```python
from build123d import *

# Parameters (mm, degrees)
BOSS_EXTRUDE1_DEPTH       = 76.2
CUT_EXTRUDE1_REACH        = 112.716
SKETCH7_R                 = 3.175
TAP_DRILL_FOR_8_32_TAP2_D = 3.4544
TAP_DRILL_FOR_8_32_TAP4_D = 3.4544
TAP_DRILL_FOR_6_32_TAP1_D = 2.7051
BOSS_EXTRUDE2_DEPTH       = 50.8


with BuildPart() as part:
    # Sketch2 → Boss-Extrude1 (new body)
    with BuildSketch(Plane.XY):
        Polygon((0, 0), (-76.2, 0), (-76.2, -25.4), (-73.025, -25.4), (-73.025, -3.175), (0, -3.175), align=None)
    extrude(amount=BOSS_EXTRUDE1_DEPTH)

    # Sketch7 → Cut-Extrude1 (cut, up to next)
    with BuildSketch(Plane.ZY.offset(76.2), mode=Mode.PRIVATE) as cut_extrude1_sk1:
        with Locations((38.1, -15.24)):
            Circle(SKETCH7_R)
    cut_extrude1_tool1 = extrude(cut_extrude1_sk1.sketch, amount=-CUT_EXTRUDE1_REACH, mode=Mode.PRIVATE) & part.part
    add(cut_extrude1_tool1.solids().sort_by_distance((-76.2, -15.24, 38.1))[0], mode=Mode.SUBTRACT)

    # Tap Drill for #8-32 Tap2 (through all)
    with Locations(Plane(origin=(0, 0, 0), x_dir=(1, 0, 0), z_dir=(0, 1, 0))):
        with Locations((-12.7, -19.05), (-12.7, -38.1), (-12.7, -57.15)):
            Hole(TAP_DRILL_FOR_8_32_TAP2_D / 2)

    # Tap Drill for #8-32 Tap4 (through all)
    with Locations(Plane(origin=(0, 0, 0), x_dir=(1, 0, 0), z_dir=(0, 1, 0))):
        with Locations((-69.028514561, -25.4), (-69.028514561, -50.8)):
            Hole(TAP_DRILL_FOR_8_32_TAP4_D / 2)

    # Tap Drill for #6-32 Tap1 (through all)
    with Locations(Plane.ZY.offset(76.2)):
        with Locations((50.8, -15.24), (63.5, -15.24)):
            Hole(TAP_DRILL_FOR_6_32_TAP1_D / 2)

    # Sketch19 → Boss-Extrude2 (add)
    with BuildSketch(Plane(origin=(0, 0, 0), x_dir=(-1, 0, 0), z_dir=(0, 0, -1))):
        Polygon((0, -3.175), (73.025, -3.175), (73.025, -25.4), (76.2, -25.4), (76.2, 0), (0, 0), align=None)
    extrude(amount=BOSS_EXTRUDE2_DEPTH)


solid = part.part
```
Check sheet for the modelled part. Datum: model origin and axes. Units: mm. A direction names the side the tool comes from. Coordinates: 2 decimals unless noted, no trailing zeros. Loops run counter-clockwise (first coordinate to the right, second up) from the corner with the lowest first, then second, coordinate; pieces in that order, holes last. Notation, with made-up numbers: M 66.25,-3.75 L 125.25,-3.75 A16 cw 125.25,1.25 Z; hole C 12.5,-11 d3. An arc over 180 degrees is marked long. Answer as a JSON object with one key per item and string values.
1. Access from +Z, -Z, +X, -X, +Y, -Y to the whole of each face (thin tool, end or side, straight path). Record for faces 5 (the flat face through (-73.025, -14, 14)), 6 (the cylindrical face through (-74.59, -15.76, 62.25)).
Outcome:
{"face 5": "+Z, -Z, +X, -Y", "face 6": "+X, -X"}
2. Sectioned sample at B-B on y = -15.24. Record the cut outline in (x, z) (3 decimals), and give its area (3 significant figures).
Outcome:
{"outline": "M -76.2,-50.8 L -73.025,-50.8 L -73.025,34.925 L -76.2,34.925 Z; M -76.2,41.275 L -73.025,41.275 L -73.025,49.447 L -76.2,49.447 Z; M -76.2,52.153 L -73.025,52.153 L -73.025,62.147 L -76.2,62.147 Z; M -76.2,64.853 L -73.025,64.853 L -73.025,76.2 L -76.2,76.2 Z", "area": "366 mm²"}
3. Release check for a two-part mould opening along Z. For faces 1 (the flat face through (-46, -1, -50.8)), 2 (the flat face through (-47, -2, 76.2)), 3 (the flat face through (-76.2, -13, 14)), 4 (the cylindrical face through (-74.635, -13.094, 35.76)) record: pulls with the +Z half, pulls with the -Z half, needs draft (parallel to the pull), parting line crosses it, or undercut.
Outcome:
{"face 1": "pulls with the -Z half", "face 2": "pulls with the +Z half", "face 3": "needs draft", "face 4": "undercut"}
4. Sectioned sample at C-C on z = 50.8. Record the cut outline in (x, y) (3 decimals).
Outcome:
{"outline": "M -76.2,-25.4 L -73.025,-25.4 L -73.025,-16.593 L -76.2,-16.593 Z; M -76.2,-13.887 L -73.025,-13.887 L -73.025,-3.175 L -70.756,-3.175 L -70.756,0 L -76.2,0 Z; M -67.301,-3.175 L 0,-3.175 L 0,0 L -67.301,0 Z"}
5. Scan lines: L1, parallel to Z at x = -12.7, y = -1.6; L2, parallel to X at y = -1.45, z = 19.05; L3, parallel to X at y = -5.75, z = 56.5 (3 decimals). Record each from-to range of solid material in increasing order. Write a range as from..to.
Outcome:
{"L1": "-50.8..17.32, 20.78..36.37, 39.83..55.42, 58.88..76.2", "L2": "-76.2..-14.43, -10.97..0", "L3": "-76.2..-73.025"}
6. Sectioned sample at D-D on x = -56.5. Record the cut outline in (y, z) (3 decimals).
Outcome:
{"outline": "M -3.175,-50.8 L 0,-50.8 L 0,76.2 L -3.175,76.2 Z"}
7. Depth check by flat-ended pin: P1, Ø10, axis at x = -58, z = 3.5, coming from the -Y side (3 decimals); P2, Ø3, axis at y = -12, z = 62, coming from the +X side (3 decimals). Enter the tip coordinate at first touch or a pass-through.
Outcome:
{"P1": "y = -3.175", "P2": "x = -73.025"}
8. Sectioned sample at A-A on z = 25.4. Record the cut outline in (x, y) (3 decimals).
Outcome:
{"outline": "M -76.2,-25.4 L -73.025,-25.4 L -73.025,-3.175 L -70.756,-3.175 L -70.756,0 L -76.2,0 Z; M -67.301,-3.175 L 0,-3.175 L 0,0 L -67.301,0 Z"}
